from build123d import *

# Parameters (mm, degrees)
SKETCH_1_R          = 37.4815
EXTRUDE_1_DEPTH     = 58
SKETCH_2_R          = 32.785
CUT_EXTRUDE_1_DEPTH = 0.5
CUT_EXTRUDE_START   = -3.23
SKETCH_3_R          = 32.785
CUT_EXTRUDE_2_DEPTH = 3.23
SKETCH_4_R          = 17.655
CUT_EXTRUDE_3_DEPTH = 79.204703724
SKETCH_5_R          = 0.766
SKETCH_5_R_2        = 0.4065
EXTRUDE_2_DEPTH     = 8.75
FILLET_1_R          = 0.5


with BuildPart() as part:
    # 草图1 → 凸台-拉伸1 (new body)
    with BuildSketch(Plane.XY):
        with Locations(Location((0, 0, 0), (0, 0, 180))):
            Circle(SKETCH_1_R)
    extrude(amount=EXTRUDE_1_DEPTH)

    # 草图2 → 切除-拉伸1 (cut)
    with BuildSketch(Plane(origin=(0, 0, 0), x_dir=(-1, 0, 0), z_dir=(0, 0, -1))):
        Circle(SKETCH_2_R)
    extrude(amount=-CUT_EXTRUDE_1_DEPTH, mode=Mode.SUBTRACT)

    # 草图3 → 切除-拉伸2 (cut)
    with BuildSketch(Plane.XY.offset(58).offset(CUT_EXTRUDE_START)):
        with Locations(Location((0, 0, 0), (0, 0, 180))):
            Circle(SKETCH_3_R)
    extrude(amount=CUT_EXTRUDE_2_DEPTH, mode=Mode.SUBTRACT)

    # 草图4 → 切除-拉伸3 (cut, through all)
    with BuildSketch(Plane(origin=(0, 0, 0.5), x_dir=(-1, 0, 0), z_dir=(0, 0, -1))):
        Circle(SKETCH_4_R)
    extrude(amount=-CUT_EXTRUDE_3_DEPTH, mode=Mode.SUBTRACT)

    # 草图5 → 凸台-拉伸2 (add)
    with BuildSketch(Plane.XY.offset(54.77)):
        with Locations((-10.715657222, 21.691015019)):
            Circle(SKETCH_5_R)
        with Locations((-6.786257081, 23.22223411)):
            Circle(SKETCH_5_R)
        with Locations((-2.650659953, 24.04785737)):
            Circle(SKETCH_5_R)
        with Locations((0, 23.9425)):
            Circle(SKETCH_5_R_2)
        with Locations((1.356512851, 24.339227635)):
            Circle(SKETCH_5_R_2)
    extrude(amount=EXTRUDE_2_DEPTH)

    # 圆角1
    fillet_1_edges = [part.edges().sort_by_distance(p)[0] for p in [
        (37.4815, 0, 0),
        (37.4815, 0, 58),
    ]]
    fillet(fillet_1_edges, radius=FILLET_1_R)


solid = part.part
For this review, take the finished solid that the model builds, in its own axes (mm). A direction names the side the tool comes from. Round coordinates to 2 decimals unless told otherwise and drop trailing zeros. Loops run counter-clockwise (first coordinate to the right, second up) from the corner with the lowest first, then second, coordinate; pieces in that order, holes last. Notation, with made-up numbers: (-12, 77.5) - (28, 77.5) arc R16 ccw to (28, 103.5) - close; hole circle Ø6 at (50, 81.5). An arc over 180 degrees is marked (long way). Put each result on its own line as item: value. Start each with the question number.
1. Mouldability with a two-part tool opening along X and no side actions: class faces 1 (the cylindrical face through (14.01, -10.743, 27.255)), 2 (the cylindrical face through (8.13, 36.59, 28.6)), 3 (the cylindrical face through (-17.63, -27.64, 56.36)), 4 (the flat face through (3, 33, 58)) as +X half, -X half, draft (parallel to the pull), parting line (faces both ways), or undercut.
2. Consider section B-B on z = 38. State the section outline as (x, y) points (1 decimal), plus the area to 3 significant figures.
3. For probe 1 along Y at (x, z) = (0, 56.6) (1 decimal); probe 2 along Y at (x, z) = (0, 21) (1 decimal); probe 3 along Z at (x, y) = (-29, 14.5), list the stretches that pass through material, from the lowest coordinate up. Write a range as [from, to].
4. Insertion check: P1, Ø1.5, axis at x = -26.5, y = 16, coming from the -Z side; P2, Ø22, axis at x = -5, y = -4.5, coming from the +Z side; P3, Ø3, axis at x = 1, z = 26.5, coming from the -Y side; P4, Ø12, axis at x = 17, y = 24.5, coming from the -Z side. Each pin has a flat end and moves straight along its axis. Give the tip position at first contact, or say it passes through.
5. Consider section A-A on y = 0. State the section outline as (x, z) points (1 decimal).
6. For faces 5 (the cylindrical face through (24.16, 22.16, 0.25)), 6 (the flat face through (-14, 14, 54.77)), 7 (the flat face through (3, 33, 0)), list the 3-axis set-ups (+Z, -Z, +X, -X, +Y, -Y) from which the entire face can be reached by the end or side of a thin tool; tool diameter is ignored.
Result sheet:
1. face 1: undercut
1. face 2: parting line
1. face 3: undercut
1. face 4: draft
2. outline: circle Ø75 at (0, 0); hole circle Ø35.3 at (0, 0)
2. area: 3,430 mm^2
3. probe 1: [-37.5, -32.8], [23.5, 24.3], [32.8, 37.5]
3. probe 2: [-37.5, -17.7], [17.7, 37.5]
3. probe 3: [0.5, 54.77]
4. P1: z = 0.5
4. P2: z = 54.77
4. P3: y = -37.48
4. P4: z = 0
5. outline: (-37.5, 0.5) arc R0.5 ccw to (-37, 0) - (-32.8, 0) - (-32.8, 0.5) - (-17.7, 0.5) - (-17.7, 54.8) - (-32.8, 54.8) - (-32.8, 58) - (-37, 58) arc R0.5 ccw to (-37.5, 57.5) - close; (17.7, 0.5) - (32.8, 0.5) - (32.8, 0) - (37, 0) arc R0.5 ccw to (37.5, 0.5) - (37.5, 57.5) arc R0.5 ccw to (37, 58) - (32.8, 58) - (32.8, 54.8) - (17.7, 54.8) - close
6. face 5: -Z
6. face 6: +Z
6. face 7: -Z, +X, -X, +Y, -Y
